For this review, take the finished solid that the model builds, in its own axes (mm). Coordinates: 2 decimals unless noted, no trailing zeros. Loops run counter-clockwise (first coordinate to the right, second up) from the corner with the lowest first, then second, coordinate; pieces in that order, holes last. Notation, with made-up numbers: (59, 41.25) - (100, 41.25) arc R23 cw to (100, 64.25) - close; hole circle Ø2 at (80, 36). An arc over 180 degrees is marked (long way). One line per item, written item: value. Start each with the question number.
1. Take a section at B-B, the plane z = 44.5. State the section outline as (x, y) points (3 decimals).
2. Take a section at C-C, the plane y = -0.5. Count the separate pieces of the cut face and the enclosed holes in it, and give its area (3 significant figures).
3. To check wall thickness, follow line 1 (Z direction, x = -21.25, y = -0.5); line 2 (Z direction, x = 21.25, y = -1.45) (3 decimals); line 3 (X direction, y = -1.4, z = -45.5). State the ranges of each line that lie inside material, in increasing order. Write a range as from..to.
4. The part is to be moulded in two halves that separate along Z. For faces 1 (the face through (0, 0, 1)), 2 (the face through (0, -1, -54.5)), 3 (the face through (23.526, -1.014, 11.352)), say which applies: released by +Z, released by -Z, zero draft, split by the parting line, or undercut.
5. Take a section at A-A, the plane x = -21.25. State the section outline as (y, z) points, and give its area (3 significant figures).
```python
from build123d import *

# Parameters (mm, degrees)
F0_W     = 60
F0_H     = 109
F1_DEPTH = 2
F2_R     = 2
F2_R_2   = 3.575
F3_DEPTH = 2
F4_R     = 2
F5_DEPTH = 2


with BuildPart() as f1:
    # F0 (on Front) → F1 (new body)
    with BuildSketch(Plane.XZ):
        Rectangle(F0_W, F0_H)
    extrude(amount=F1_DEPTH)

    # F2 (on face) → F3 (cut, through all)
    with BuildSketch(Plane.XZ.offset(2)):
        with Locations((-21.25, 44.5)):
            Circle(F2_R)
        with Locations((-21.25, -44.5)):
            Circle(F2_R)
        with Locations((21.25, 44.5)):
            Circle(F2_R_2)
        with Locations((21.25, -44.5)):
            Circle(F2_R_2)
    extrude(amount=-F3_DEPTH, mode=Mode.SUBTRACT)

    # F4 (on face) → F5 (cut, through all)
    with BuildSketch(Plane.XZ.offset(2)):
        with Locations((-25, 10)):
            Circle(F4_R)
        with Locations((25, 10)):
            Circle(F4_R)
        with Locations((-25, -10)):
            Circle(F4_R)
        with Locations((25, -10)):
            Circle(F4_R)
    extrude(amount=-F5_DEPTH, mode=Mode.SUBTRACT)


solid = f1.part
```
Solutions:
1. outline: (-30, -2) - (-23.25, -2) - (-23.25, 0) - (-30, 0) - close; (-19.25, -2) - (17.675, -2) - (17.675, 0) - (-19.25, 0) - close; (24.825, -2) - (30, -2) - (30, 0) - (24.825, 0) - close
2. separate pieces: 1
2. enclosed holes: 8
2. area: 6,380 mm2
3. line 1: -54.5..-46.5, -42.5..42.5, 46.5..54.5
3. line 2: -54.5..-48.075, -40.925..40.925, 48.075..54.5
3. line 3: -30..-22.98, -19.52..17.82, 24.68..30
4. face 1: zero draft
4. face 2: released by -Z
4. face 3: undercut
5. outline: (-2, -54.5) - (0, -54.5) - (0, -46.5) - (-2, -46.5) - close; (-2, -42.5) - (0, -42.5) - (0, 42.5) - (-2, 42.5) - close; (-2, 46.5) - (0, 46.5) - (0, 54.5) - (-2, 54.5) - close
5. area: 202 mm2
